```python
from build123d import *
from build123d.topology import SkipClean

# Parameters (mm, degrees)
SKETCH1_R                = 10
SKETCH1_R_2              = 6
BOSS_EXTRUDE1_DEPTH      = 40
BOSS_EXTRUDE4_DEPTH      = 3
BOSS_EXTRUDE4_DEPTH_BACK = 4
SKETCH7_R                = 20
FILLET3_R                = 6
SKETCH8_R                = 15
CUT_EXTRUDE3_DEPTH       = 2


with BuildPart() as part:
    # Sketch1 → Boss-Extrude1 (new body)
    with BuildSketch(Plane.XY):
        Circle(SKETCH1_R)
        Circle(SKETCH1_R_2, mode=Mode.SUBTRACT)
    extrude(amount=BOSS_EXTRUDE1_DEPTH)

    # Sketch6 → Revolve1 (revolve)
    with BuildSketch(Plane(origin=(0, 0, 0), x_dir=(1, 0, 0), z_dir=(0, 1, 0))):
        with BuildLine():
            Line((-10, 0), (0, 0))
            Line((0, 0), (0, 10))
            ThreePointArc((0, 10), (-7.071067812, 7.071067812), (-10, 0))
        make_face()
    revolve(axis=Axis((0, 0, -10), (0, 0, 1)))

    # Sketch7 → Boss-Extrude4 (add, two sides: drawn at the far end of the back side and taken through both)
    with SkipClean():  # the faces are left unmerged after this step: merging them gives an invalid solid
        with BuildSketch(Plane.ZY.offset(10).offset(-BOSS_EXTRUDE4_DEPTH_BACK)):
            with Locations((20, 0)):
                Circle(SKETCH7_R)
        extrude(amount=BOSS_EXTRUDE4_DEPTH + BOSS_EXTRUDE4_DEPTH_BACK)

    # Fillet3
    fillet3_edges = [part.edges().sort_by_distance(p)[0] for p in [
        (-6, 8, 20),
        (-6, -8, 20),
    ]]
    fillet(fillet3_edges, radius=FILLET3_R)

    # Sketch8 → Cut-Extrude3 (cut)
    with BuildSketch(Plane.ZY.offset(13)):
        with Locations((20, 0)):
            Circle(SKETCH8_R)
    extrude(amount=-CUT_EXTRUDE3_DEPTH, mode=Mode.SUBTRACT)


solid = part.part
```
Work out the finished part from the listing and answer in its coordinate system (mm). A direction names the side the tool comes from. Give positions to 0.01 mm unless a question says otherwise; leave off trailing zeros. Loops run counter-clockwise (first coordinate to the right, second up) from the corner with the lowest first, then second, coordinate; pieces in that order, holes last. Notation, with made-up numbers: (38, 41.25) - (48, 41.25) arc R19 ccw to (48, 66.25) - close; hole circle Ø6 at (-33.75, 67). An arc over 180 degrees is marked (long way). Use CSV: the item, a comma, the result in double quotes. Start each with the question number.
(1) Find section D-D, the plane z = 11. Determine the outline of the cut face in (x, y).
(2) Determine the mould class of faces 4 (the face through (-4.196, -11.711, 19.758)), 5 (the face through (-11, 0, 20)), 6 (the face through (-6, 18, 20)) for opening direction Y: released by +Y, released by -Y, zero draft, split by the parting line, or undercut.
(3) Find the intervals of material crossed by L1, parallel to Y at x = -12.15, z = 20; L2, parallel to X at y = 0, z = 13.5; L3, parallel to Y at x = 2.5, z = 35.5, in increasing order.
(4) Find section A-A, the plane z = 20. Determine the outline of the cut face in (x, y).
(5) Find section B-B, the plane x = 1.25. Determine the outline of the cut face in (y, z), plus the area to 3 significant figures.
(6) A tool of negligible diameter and unlimited length cuts with its end or side. For faces 1 (the face through (-6, 0, 20)), 2 (the face through (-6, -18, 20)), 3 (the face through (-12.014, 0.66, 5.015)), from which of +Z, -Z, +X, -X, +Y, -Y can it reach the whole face along a straight path? Write none if from no direction.
(7) Each of these flat-tipped pins is pushed along its axis until it touches: pin 1 (4 mm diameter, centred on y = 15.5, z = 3, fed in from +X); pin 2 (7 mm diameter, centred on x = 0, y = 0, fed in from +Z); pin 3 (1 mm diameter, centred on x = -8, y = -3, fed in from -Z); pin 4 (1.5 mm diameter, centred on x = -7, z = 23.5, fed in from -Y). Where does it stop, or does it pass through?
(8) Find section C-C, the plane y = 8. Determine the outline of the cut face in (x, z).
Results found:
1,outline,"(-13, -17.86) - (-6, -17.86) - (-6, -16) arc R6 cw to (0, -10) arc R10 ccw to (0, 10) arc R6 cw to (-6, 16) - (-6, 17.86) - (-13, 17.86) - (-13, 12) - (-11, 12) - (-11, -12) - (-13, -12) - close; hole circle Ø12 at (0, 0)"
2,face 4,"released by -Y"
2,face 5,"undercut"
2,face 6,"zero draft"
3,L1,"-20 to -15, 15 to 20"
3,L2,"-11 to -6, 6 to 10"
3,L3,"-9.68 to -5.45, 5.45 to 9.68"
4,outline,"(-13, -20) - (-6, -20) - (-6, -16) arc R6 cw to (0, -10) arc R10 ccw to (0, 10) arc R6 cw to (-6, 16) - (-6, 20) - (-13, 20) - (-13, 15) - (-11, 15) - (-11, -15) - (-13, -15) - close; hole circle Ø12 at (0, 0)"
5,outline,"(-9.92, 0) arc R9.92 ccw to (9.92, 0) - (9.92, 40) - (5.87, 40) - (5.87, 0) - (-5.87, 0) - (-5.87, 40) - (-9.92, 40) - close"
5,area,"479 mm^2"
6,face 1,"+Z"
6,face 2,"+Z, -Z, +X, -Y"
6,face 3,"-X"
7,pin 1,"through"
7,pin 2,"z = 0"
7,pin 3,"z = -5.94"
7,pin 4,"y = -19.81"
8,outline,"(-13, 1.67) - (-6, 1.67) - (-6, 0) arc R6 ccw to (6, 0) - (6, 40) - (-6, 40) - (-6, 38.33) - (-13, 38.33) - (-13, 32.69) - (-11, 32.69) - (-11, 7.31) - (-13, 7.31) - close"
